```python
from build123d import *

# Parameters (mm, degrees)
F2_R          = 3
F3_DEPTH      = 9.001
F3_DEPTH_BACK = 9.001


with BuildPart() as f1:
    # F0 (on Front) → F1 (revolve)
    with BuildSketch(Plane.XZ):
        Polygon((0, 6), (0, 0), (138, 0), (138, 9), (114, 9), (114, 6), (104, 6), (104, 8), (22, 8), (22, 6), (13, 6), (13, 4), (7, 4), (7, 6), align=None)
    revolve(axis=Axis((69, 0, 0), (-1, 0, 0)))

    # F2 (on Top) → F3 (cut, two sides)
    with BuildSketch(Plane.XY) as f3_sk:
        with Locations((126, 0)):
            Circle(F2_R)
    extrude(amount=-F3_DEPTH, mode=Mode.SUBTRACT)
    extrude(f3_sk.sketch, amount=F3_DEPTH_BACK, mode=Mode.SUBTRACT)


solid = f1.part
```
For this review, take the finished solid that the model builds, in its own axes (mm). A direction names the side the tool comes from. Coordinates: 2 decimals unless noted, no trailing zeros. Loops run counter-clockwise (first coordinate to the right, second up) from the corner with the lowest first, then second, coordinate; pieces in that order, holes last. Notation, with made-up numbers: (10, 58) - (16, 58) arc R7 ccw to (16, 71) - close; hole circle Ø10 at (32, -4). An arc over 180 degrees is marked (long way). Use one line per item in the form item = value. Start each with the question number.
1) For faces 4 (the face through (3, 0, -6)), 5 (the face through (0, 0, 0)), 6 (the face through (7, -3.92, 1.42)), list the 3-axis set-ups (+Z, -Z, +X, -X, +Y, -Y) from which the entire face can be reached by the end or side of a thin tool; tool diameter is ignored.
2) Draft analysis for pull direction X (two halves, no side actions). For faces 1 (the face through (17, 0, -6)), 2 (the face through (138, 0, 0)), 3 (the face through (13, -3.92, -1.42)), state which applies: released by +X, released by -X, zero draft, split by the parting line, or undercut.
3) To check wall thickness, follow probe 1 along X at (y, z) = (5.75, 5.5); probe 2 along X at (y, z) = (0.25, -1.75); probe 3 along X at (y, z) = (-2.75, 3.75). State the ranges of each line that lie inside material, in increasing order. Write a range as from..to.
4) Take a section at C-C (x = 126). State the section outline as (y, z) points, plus the area to 3 significant figures.
5) For pin 1 (8 mm diameter, centred on x = 93, y = 3, fed in from +Z); pin 2 (6 mm diameter, centred on x = 45, y = -5.5, fed in from -Z); pin 3 (2 mm diameter, centred on x = 115.5, y = 3, fed in from -Z), all flat-tipped, find the tip position at first contact; note any pin that passes through.
6) Take a section at A-A (y = 0). State the section outline as (x, z) points, plus the area to 3 significant figures.
7) Take a section at B-B (x = 110). State the section outline as (y, z) points.
From the geometry:
q1.face_4 = -X
q1.face_5 = +Z, -Z, -X, +Y, -Y
q1.face_6 = none
q2.face_1 = zero draft
q2.face_2 = released by +X
q2.face_3 = undercut
q3.probe_1 = 22..104, 114..138
q3.probe_2 = 0..123.01, 128.99..138
q3.probe_3 = 0..7, 13..124.8, 127.2..138
q4.outline = (-3, -8.49) - (-3, 8.49) arc R9 ccw to start; (3, -8.49) arc R9 ccw to (3, 8.49) - close
q4.area = 149 mm2
q5.pin_1 = 8
q5.pin_2 = -7.6
q5.pin_3 = -8.77
q6.outline = (0, -6) - (7, -6) - (7, -4) - (13, -4) - (13, -6) - (22, -6) - (22, -8) - (104, -8) - (104, -6) - (114, -6) - (114, -9) - (123, -9) - (123, 9) - (114, 9) - (114, 6) - (104, 6) - (104, 8) - (22, 8) - (22, 6) - (13, 6) - (13, 4) - (7, 4) - (7, 6) - (0, 6) - close; (129, -9) - (138, -9) - (138, 9) - (129, 9) - close
q6.area = 2,000 mm2
q7.outline = circle Ø12 at (0, 0)
